Geometry check sheet. Reference: the model listing, model coordinates, mm. A direction names the side the tool comes from. Coordinates: 2 decimals unless noted, no trailing zeros. Order: outer loops, then holes, each group sorted by start corner. A loop starts at its lowest first (then second) coordinate and runs counter-clockwise, first axis right, second up. Notation, with made-up numbers: (-13.5, 9.25) - (19.5, 9.25) arc R28 cw to (19.5, 35.25) - close; hole circle Ø7 at (-6, 32). An arc over 180 degrees is marked (long way). Return JSON: item names as keys, results as strings. Group by question number.
Item 1: Gauge pin test, flat ends, axial feed: pin 1 (20.5 mm diameter, centred on x = 0, z = 0, fed in from +Y); pin 2 (2.5 mm diameter, centred on x = 20.32, y = 4.76, fed in from -Z); pin 3 (2.5 mm diameter, centred on x = -20.32, y = 4.76, fed in from +Z). Record the tip position at first contact, or that the pin passes through.
Item 2: Section check A-A on x = 0. Enter the section's corners in (y, z) (1 decimal).
Item 3: Tool access check on faces 5 (the cylindrical face through (18.32, 5.03, 33.78)), 6 (the cylindrical face through (-7.7, 1.8, 10.1)), 7 (the cylindrical face through (-18.35, 5.2, -33.78)). Record the directions out of +Z, -Z, +X, -X, +Y, -Y that give a thin tool (end or side, any length) a straight path to the whole face; none if there is none.
Item 4: Section check D-D on z = 9. Enter the section's corners in (x, y) (3 decimals), then the cut area to 3 significant figures.
Item 5: Scan lines: probe 1 along X at (y, z) = (4.25, 0.5); probe 2 along Y at (x, z) = (-20.32, 35.5) (3 decimals); probe 3 along Z at (x, y) = (-4, 1.5). Record each from-to range of solid material in increasing order.
Item 6: Section check C-C on y = 1.5. Enter the section's corners in (x, z).
Item 7: Draft check along X on faces 1 (the cylindrical face through (18.32, 5.03, -33.78)), 2 (the flat face through (0, 5, 36.908)), 3 (the flat face through (26.67, 5, 1)), 4 (the flat face through (-26.67, 5, 1)). Enter one of: pulls with the +X half, pulls with the -X half, needs draft (parallel to the pull), parting line crosses it, or undercut.
Item 8: Section check B-B on z = 0. Enter the section's corners in (x, y) (1 decimal).
from build123d import *

# Parameters (mm, degrees)
SKETCH2_W                           = 53.34
SKETCH2_H                           = 73.816694632
SKETCH2_R                           = 7.14375
BOSS_EXTRUDE1_DEPTH                 = 9.525
SKETCH3_R                           = 11.1125
CUT_EXTRUDE1_DEPTH                  = 0.79375
SKETCH4_R                           = 12.7
CUT_EXTRUDE2_DEPTH                  = 3.571875
TAP_DRILL_FOR_10_32_TAP1_AT_2_COUNT = 2
TAP_DRILL_FOR_10_32_TAP1_AT_2_PITCH = 40.64
TAP_DRILL_FOR_10_32_TAP2_D          = 4.0386


with BuildPart() as part:
    # Sketch2 → Boss-Extrude1 (new body)
    with BuildSketch(Plane(origin=(0, 0, 0), x_dir=(1, 0, 0), z_dir=(0, 1, 0))):
        Rectangle(SKETCH2_W, SKETCH2_H)
        with Locations(Location((0, 0, 0), (0, 0, 90))):
            Circle(SKETCH2_R, mode=Mode.SUBTRACT)
    extrude(amount=BOSS_EXTRUDE1_DEPTH)

    # Sketch3 → Cut-Extrude1 (cut)
    with BuildSketch(Plane(origin=(0, 9.525, 0), x_dir=(1, 0, 0), z_dir=(0, 1, 0))):
        with Locations(Location((0, 0, 0), (0, 0, 270))):
            Circle(SKETCH3_R)
    extrude(amount=-CUT_EXTRUDE1_DEPTH, mode=Mode.SUBTRACT)

    # Sketch4 → Cut-Extrude2 (cut)
    with BuildSketch(Plane.XZ):
        with Locations(Location((0, 0, 0), (0, 0, 270))):
            Circle(SKETCH4_R)
    extrude(amount=-CUT_EXTRUDE2_DEPTH, mode=Mode.SUBTRACT)

    # Sketch6 → Tap Drill for #10-32 Tap1 (revolve, cut)
    with BuildSketch(Plane(origin=(-20.32, 4.7625, 36.908347316), x_dir=(0, -1, 0), z_dir=(1, 0, 0))):
        Polygon((0, 0), (0, 7.563317848), (2.0193, 6.35), (2.0193, 0), align=None)
    tap_drill_for_10_32_tap1 = revolve(axis=Axis((-20.32, 4.7625, 43.258347316), (0, 0, -1)), mode=Mode.SUBTRACT)

    # Tap Drill for #10-32 Tap1 at 2: Tap Drill for #10-32 Tap1 ×2
    with Locations(*[(i * TAP_DRILL_FOR_10_32_TAP1_AT_2_PITCH, 0, 0) for i in range(1, TAP_DRILL_FOR_10_32_TAP1_AT_2_COUNT)]):
        add(tap_drill_for_10_32_tap1, mode=Mode.SUBTRACT)

    # Mirror1: Tap Drill for #10-32 Tap1 across plane
    add(tap_drill_for_10_32_tap1.mirror(Plane.XY), mode=Mode.SUBTRACT)

    # Mirror1 copy 1 sketch → Mirror1 copy 1 (revolve, cut)
    with BuildSketch(Plane(origin=(20.32, 4.7625, -36.908347316), x_dir=(0, -1, 0), z_dir=(1, 0, 0))):
        Polygon((0, 0), (0, -7.563317848), (2.0193, -6.35), (2.0193, 0), align=None)
    revolve(axis=Axis((20.32, 4.7625, -43.258347316), (0, 0, -1)), mode=Mode.SUBTRACT)

    # Tap Drill for #10-32 Tap2 (through all)
    with Locations(Plane(origin=(0, 9.525, 0), x_dir=(1, 0, 0), z_dir=(0, 1, 0))):
        with Locations((-20.622229928, 11.90625), (-20.622229928, -11.90625), (20.622229928, -11.90625), (20.622229928, 11.90625)):
            Hole(TAP_DRILL_FOR_10_32_TAP2_D / 2)


solid = part.part
Computed:
{
 "1": {"pin 1": "stops at y = 8.73", "pin 2": "stops at z = -30.1", "pin 3": "stops at z = 30.1"},
 "2": {"outline": "(0, -36.9) - (9.5, -36.9) - (9.5, -11.1) - (8.7, -11.1) - (8.7, -7.1) - (3.6, -7.1) - (3.6, -12.7) - (0, -12.7) - close; (0, 12.7) - (3.6, 12.7) - (3.6, 7.1) - (8.7, 7.1) - (8.7, 11.1) - (9.5, 11.1) - (9.5, 36.9) - (0, 36.9) - close"},
 "3": {"face 5": "+Z", "face 6": "-Y", "face 7": "-Z"},
 "4": {"outline": "(-26.67, 0) - (-8.96, 0) - (-8.96, 3.572) - (8.96, 3.572) - (8.96, 0) - (26.67, 0) - (26.67, 9.525) - (6.518, 9.525) - (6.518, 8.731) - (-6.518, 8.731) - (-6.518, 9.525) - (-26.67, 9.525) - close", "area": "434 mm²"},
 "5": {"probe 1": "x = -26.67 to -7.13, 7.13 to 26.67", "probe 2": "y = 0 to 2.743, 6.782 to 9.525", "probe 3": "z = -36.91 to -12.05, 12.05 to 36.91"},
 "6": {"outline": "(-26.67, -36.91) - (26.67, -36.91) - (26.67, 36.91) - (-26.67, 36.91) - close; hole circle Ø4.04 at (-20.62, -11.91); hole circle Ø4.04 at (-20.62, 11.91); hole circle Ø25.4 at (0, 0); hole circle Ø4.04 at (20.62, -11.91); hole circle Ø4.04 at (20.62, 11.91)"},
 "7": {"face 1": "undercut", "face 2": "needs draft", "face 3": "pulls with the +X half", "face 4": "pulls with the -X half"},
 "8": {"outline": "(-26.7, 0) - (-12.7, 0) - (-12.7, 3.6) - (-7.1, 3.6) - (-7.1, 8.7) - (-11.1, 8.7) - (-11.1, 9.5) - (-26.7, 9.5) - close; (7.1, 3.6) - (12.7, 3.6) - (12.7, 0) - (26.7, 0) - (26.7, 9.5) - (11.1, 9.5) - (11.1, 8.7) - (7.1, 8.7) - close"}
}
